from build123d import *

# Parameters (mm, degrees)
CUT_EXTRUDE1_DEPTH       = 29.014947405
BOSS_EXTRUDE1_START      = 13.11
BOSS_EXTRUDE1_OUTLINE_R  = 7.478502705
BOSS_EXTRUDE1_DEPTH      = 10.08
CIRPATTERN1_COUNT        = 3
BOSS_EXTRUDE2_DEPTH      = 10.08
BOSS_EXTRUDE2_DEPTH_BACK = 265
SKETCH6_R                = 9


# Read off the part's stored shape, not the designer's step: Boss-Extrude1, Revolve3
with BuildPart() as part:
    # Sketch1 → Revolve1 (revolve)
    with BuildSketch(Plane.XY):
        with BuildLine():
            Line((-8.653846154, 12.951890954), (-8.653846154, 9))
            Line((-8.653846154, 9), (8.653846154, 9))
            Line((8.653846154, 9), (8.653846154, 12.951890954))
            ThreePointArc((8.653846154, 12.951890954), (0, 15.576923077), (-8.653846154, 12.951890954))
        make_face()
    revolve(axis=Axis((-47.061566383, 0, 0), (1, 0, 0)))

    # Sketch2 → Cut-Extrude1 (cut, symmetric)
    with BuildSketch(Plane(origin=(8.653846154, 0, 0), x_dir=(0, 0, -1), z_dir=(1, 0, 0))):
        Polygon((-17.183661108, 13.11), (20.1337897, 13.11), (18.772985043, 23.764289573), (-17.183661108, 23.764289573), align=None)
    cut_extrude1 = extrude(amount=CUT_EXTRUDE1_DEPTH, both=True, mode=Mode.SUBTRACT)

    # Boss-Extrude1 outline → Boss-Extrude1 (add)
    with BuildSketch(Plane(origin=(0, 0, 0), x_dir=(1, 0, 0), z_dir=(0, 1, 0)).offset(BOSS_EXTRUDE1_START)):
        Circle(BOSS_EXTRUDE1_OUTLINE_R)
    boss_extrude1 = extrude(amount=BOSS_EXTRUDE1_DEPTH)

    # Sketch4 → Revolve2 (revolve)
    with BuildSketch(Plane(origin=(0, 0, 0), x_dir=(0, 0, -1), z_dir=(1, 0, 0)), mode=Mode.PRIVATE) as revolve2_sk:
        with BuildLine():
            Line((7.478502705, 25.422863672), (7.478502705, 23.19))
            Line((7.478502705, 23.19), (0, 23.19))
            Line((0, 23.19), (0, 26.5))
            ThreePointArc((0, 26.5), (3.777837522, 26.229333649), (7.478502705, 25.422863672))
        make_face()
    revolve2 = revolve(revolve2_sk.sketch.rotate(Axis((0, 0, 0), (0, 1, 0)), 180), axis=Axis((0, 0, 0), (0, 1, 0)))

    # Revolve3 outline → Revolve3 (revolve)
    with BuildSketch(Plane.XY):
        with BuildLine():
            Line((7.478502705, 13.109999994), (12.254015665, 13.109999994))
            ThreePointArc((12.254015665, 13.109999994), (13.25, 18.15), (12.254015665, 23.190000006))
            Line((12.254015665, 23.190000006), (7.478502705, 23.19))
            Line((7.478502705, 23.19), (7.478502705, 13.109999994))
        make_face()
    revolve3 = revolve(axis=Axis((0, 0, 0), (0, 1, 0)))

    # CirPattern1: Cut-Extrude1, Boss-Extrude1, Revolve2, Revolve3 ×3 about axis
    cirpattern1_axis = Axis((0, 0, 0), (1, 0, 0))
    add([cut_extrude1.rotate(cirpattern1_axis, i * 360 / CIRPATTERN1_COUNT) for i in range(1, CIRPATTERN1_COUNT)], mode=Mode.SUBTRACT)
    add([boss_extrude1.rotate(cirpattern1_axis, i * 360 / CIRPATTERN1_COUNT) for i in range(1, CIRPATTERN1_COUNT)])
    add([revolve2.rotate(cirpattern1_axis, i * 360 / CIRPATTERN1_COUNT) for i in range(1, CIRPATTERN1_COUNT)])
    add([revolve3.rotate(cirpattern1_axis, i * 360 / CIRPATTERN1_COUNT) for i in range(1, CIRPATTERN1_COUNT)])

    # Sketch6 → Boss-Extrude2 (add, two sides: drawn at the far end of the back side and taken through both)
    with BuildSketch(Plane.ZY.offset(8.653846154).offset(-BOSS_EXTRUDE2_DEPTH_BACK)):
        Circle(SKETCH6_R)
    extrude(amount=BOSS_EXTRUDE2_DEPTH + BOSS_EXTRUDE2_DEPTH_BACK)


solid = part.part
Verification items for the finished model (mm, model axes). A direction names the side the tool comes from. Coordinates: 2 decimals unless noted, no trailing zeros. Order: outer loops, then holes, each group sorted by start corner. A loop starts at its lowest first (then second) coordinate and runs counter-clockwise, first axis right, second up. Notation, with made-up numbers: (38, 53) -> (48, 53) arc R28 cw to (48, 84) -> close; hole circle Ø9 at (48, 63.25). An arc over 180 degrees is marked (long way). Use CSV: the item, a comma, the result in double quotes. Start each with the question number.
Q1. Section check C-C, the plane y = 16. Record the cut outline in (x, z), and give its area (3 significant figures).
Q2. Section check A-A, the plane z = 0. Record the cut outline in (x, y).
Q3. Tool access check on faces 4 (the flat face through (-2.6, 13.11, -8.3)), 5 (the flat face through (-6, 23.19, 5)), 6 (the flat face through (-8.654, -9, -3)). Record the directions out of +Z, -Z, +X, -X, +Y, -Y that give a thin tool (end or side, any length) a straight path to the whole face; none if there is none.
Q4. Section check B-B, the plane x = 48. Record the cut outline in (y, z), and give its area (3 significant figures).
Q5. Thickness scan on line 1 along X through (y, z) = (-1.5, 12); line 2 along Z through (x, y) = (17, -5); line 3 along Y through (x, z) = (133.5, 8). Record the ranges inside material, lowest first.
Q6. Draft check along Z on faces 1 (the flat face through (-18.734, 0, 0)), 2 (the cylindrical face through (-7.3, 24.29, -1.62)), 3 (the flat face through (-2.55, -13.78, -7.18)). Enter one of: +Z half, -Z half, draft (parallel to the pull), parting line (faces both ways), or undercut.
Q7. Depth check by flat-ended pin: P1, Ø1.5, axis at y = -10, z = -1.5, coming from the +X side; P2, Ø12.5, axis at x = 5.5, z = 5.5, coming from the -Y side; P3, Ø4, axis at y = 17, z = 14, coming from the -X side. Enter the tip coordinate at first touch or a pass-through.
Returned:
1,outline,"circle Ø26.15 at (0, 0)"
1,area,"537 mm^2"
2,outline,"(-18.73, -9) -> (-8.65, -9) -> (-8.65, -12.95) arc R15.58 ccw to (8.65, -12.95) -> (8.65, -9) -> (256.35, -9) -> (256.35, 9) -> (8.65, 9) -> (8.65, 12.95) arc R15.58 ccw to (8.41, 13.11) -> (12.25, 13.11) arc R13.25 ccw to (12.25, 23.19) -> (7.48, 23.19) -> (7.48, 25.42) arc R26.5 ccw to (-7.48, 25.42) -> (-7.48, 23.19) -> (-12.25, 23.19) arc R13.25 ccw to (-12.25, 13.11) -> (-8.41, 13.11) arc R15.58 ccw to (-8.65, 12.95) -> (-8.65, 9) -> (-18.73, 9) -> close"
3,face 4,"none"
3,face 5,"+Y"
3,face 6,"-X"
4,outline,"circle Ø18 at (0, 0)"
4,area,"254 mm^2"
5,line 1,"x = -8.65 to 8.65"
5,line 2,"z = -7.48 to 7.48"
5,line 3,"y = -4.12 to 4.12"
6,face 1,"draft"
6,face 2,"parting line"
6,face 3,"undercut"
7,P1,"stops at x = 8.65"
7,P2,"stops at y = -21.19"
7,P3,"stops at x = -5.52"
